Could you check a few things on this model? Use its own coordinates, in mm. Coordinates: 2 decimals unless noted, no trailing zeros. Loops run counter-clockwise (first coordinate to the right, second up) from the corner with the lowest first, then second, coordinate; pieces in that order, holes last. Notation, with made-up numbers: (2.25, -12) - (58.25, -12) arc R11 ccw to (58.25, 0) - close; hole circle Ø7 at (71, 64). An arc over 180 degrees is marked (long way). Put each result on its own line as item: value. Start each with the question number.
```python
from build123d import *

# Parameters (mm, degrees)
F0_R     = 23.71864
F1_DEPTH = 25.4
F2_SIZE2 = 5.08
F2_SIZE  = 5.08


with BuildPart() as f1:
    # F0 (on Top) → F1 (new body)
    with BuildSketch(Plane.XY):
        with BuildLine():
            Line((-35.99517, -62.541589), (35.99517, -62.541589))
            Line((35.99517, -62.541589), (35.99517, 56.191589))
            ThreePointArc((35.99517, 56.191589), (34.135299, 60.681717), (29.64517, 62.541589))
            Line((29.64517, 62.541589), (-29.64517, 62.541589))
            ThreePointArc((-29.64517, 62.541589), (-34.135299, 60.681717), (-35.99517, 56.191589))
            Line((-35.99517, 56.191589), (-35.99517, -62.541589))
        make_face()
        Circle(F0_R, mode=Mode.SUBTRACT)
    extrude(amount=F1_DEPTH)

    # F2
    f2_edges = [f1.edges().sort_by_distance(p)[0] for p in [
        (-35.99517, -3.175, 25.4),
        (0, -62.541589, 25.4),
        (35.99517, -3.175, 25.4),
        (34.135299, 60.681717, 25.4),
        (0, 62.541589, 25.4),
        (-34.135299, 60.681717, 25.4),
        (-23.71864, 0, 25.4),
    ]]
    chamfer(f2_edges, length=F2_SIZE, length2=F2_SIZE2)


solid = f1.part
```
(1) If we mould it in two halves opening along X, with no side actions, what happens to faces 1 (the conical face through (-3.1, 23.8, 20.6)), 2 (the cylindrical face through (34.184, 60.632, 10.018)), 3 (the flat face through (-1, -62.542, 10))? For each: pulls with the +X half, pulls with the -X half, needs draft (parallel to the pull), parting line crosses it, or undercut.
(2) I need wall thicknesses on L1, parallel to Y at x = 0, z = 6; L2, parallel to X at y = 3.5, z = 21.25; L3, parallel to Y at x = 11, z = 11.5. Which ranges of each line are inside material? Lowest first, please. Write a range as [from, to].
(3) I want a section at B-B on x = 0. List the corners of the cut face in (y, z) for me, and give its area (3 significant figures).
(4) I want a section at A-A on y = 0. List the corners of the cut face in (x, z) for me, and give its area (3 significant figures).
(5) For pin 1 Ø1.5 at (x, z) = (-24.5, 21.5) entering from +Y, with a flat end and sliding along its axis, tell me the tip position at first contact or that it passes through.
(6) I want a section at C-C on z = 11.5. List the corners of the cut face in (x, y) for me, and give its area (3 significant figures).
Answer sheet:
1. face 1: undercut
1. face 2: pulls with the +X half
1. face 3: needs draft
2. L1: y = [-62.54, -23.72], [23.72, 62.54]
2. L2: x = [-35.07, -24.4], [24.4, 35.07]
2. L3: y = [-62.54, -21.01], [21.01, 62.54]
3. outline: (-62.54, 0) - (-23.72, 0) - (-23.72, 20.32) - (-28.8, 25.4) - (-57.46, 25.4) - (-62.54, 20.32) - close; (23.72, 0) - (62.54, 0) - (62.54, 20.32) - (57.46, 25.4) - (28.8, 25.4) - (23.72, 20.32) - close
3. area: 1,920 mm^2
4. outline: (-36, 0) - (-23.72, 0) - (-23.72, 20.32) - (-28.8, 25.4) - (-30.92, 25.4) - (-36, 20.32) - close; (23.72, 0) - (36, 0) - (36, 20.32) - (30.92, 25.4) - (28.8, 25.4) - (23.72, 20.32) - close
4. area: 572 mm^2
5. pin 1: stops at y = 62.11
6. outline: (-36, -62.54) - (36, -62.54) - (36, 56.19) arc R6.35 ccw to (29.65, 62.54) - (-29.65, 62.54) arc R6.35 ccw to (-36, 56.19) - close; hole circle Ø47.44 at (0, 0)
6. area: 7,220 mm^2
